```python
from build123d import *

# Parameters (mm, degrees)
F3_R     = 2.5
F4_DEPTH = 76.2


with BuildPart() as f2:
    # F0 (on Front) → F2 (revolve)
    with BuildSketch(Plane.XZ):
        with BuildLine():
            Line((-42, 11.43), (-42, 0))
            Line((-42, 0), (-40, 0))
            Line((-40, 0), (-40, 11.43))
            ThreePointArc((-40, 11.43), (-40.957761, 13.742239), (-43.27, 14.7))
            Line((-43.27, 14.7), (-46, 14.7))
            Line((-46, 14.7), (-46, 94.7))
            Line((-46, 94.7), (-4, 94.7))
            Line((-4, 94.7), (-4, 93.2))
            Line((-4, 93.2), (-4.4, 93.2))
            Line((-4.4, 93.2), (-4, 89.7))
            Line((-4, 89.7), (-4.4, 89.7))
            Line((-4.4, 89.7), (-4, 86.2))
            Line((-4, 86.2), (-2.5, 86.2))
            Line((-2.5, 86.2), (-2.5, 96.7))
            Line((-2.5, 96.7), (-47.365, 96.7))
            ThreePointArc((-47.365, 96.7), (-47.814013, 96.514013), (-48, 96.065))
            Line((-48, 96.065), (-48, 13.97))
            ThreePointArc((-48, 13.97), (-47.628026, 13.071974), (-46.73, 12.7))
            Line((-46.73, 12.7), (-43.27, 12.7))
            ThreePointArc((-43.27, 12.7), (-42.371974, 12.328026), (-42, 11.43))
        make_face()
    revolve(axis=Axis((0, 0, 51.843766), (0, 0, 1)))

    # F3 (on Front) → F4 (cut)
    with BuildSketch(Plane.XZ):
        with Locations((6.35, 43.18)):
            Circle(F3_R)
    extrude(amount=F4_DEPTH, mode=Mode.SUBTRACT)

    # F7 (on offset) → F8 (revolve)
    with BuildSketch(Plane.YZ.offset(6.35)):
        Polygon((-42.69981, 47.18), (-46.19981, 47.18), (-46.19981, 45.68), (-35.69981, 45.68), (-35.69981, 47.18), (-39.19981, 47.18), align=None)
        Polygon((-42.69981, 47.58), (-42.69981, 47.18), (-39.19981, 47.18), align=None)
        Polygon((-39.19981, 47.58), (-39.19981, 47.18), (-35.69981, 47.18), align=None)
    revolve(axis=Axis((6.35, -16.508139, 43.18), (0, 1, 0)))


solid = f2.part
```
Check sheet for the modelled part. Datum: model origin and axes. Units: mm. A direction names the side the tool comes from. Give positions to 0.01 mm unless a question says otherwise; leave off trailing zeros. Loops run counter-clockwise (first coordinate to the right, second up) from the corner with the lowest first, then second, coordinate; pieces in that order, holes last. Notation, with made-up numbers: M 45,61.25 L 70,61.25 A31 cw 70,97.25 Z; hole C -28,37.5 d10. An arc over 180 degrees is marked long. Answer in a Markdown table with one row per item.
1) Mould release check, pull along Y, two halves, no side actions. Record for faces 1 (the face through (0.867, 3.905, 93.94)), 2 (the face through (-37.1, 15.4, 0)), 3 (the face through (10.405, 46.859, 54.443)): released by +Y, released by -Y, zero draft, split by the parting line, or undercut.
Solutions:
| item | result |
|---|---|
| face 1 | undercut |
| face 2 | zero draft |
| face 3 | split by the parting line |
2) Cross-section at A-A (z = 75). Enter the section's corners in (x, y).
Solutions:
| item | result |
|---|---|
| outline | C 0,0 d96; hole C 0,0 d92 |
3) Cross-section at B-B (z = 43.18). Enter the section's corners in (x, y), plus the area to 3 significant figures.
Solutions:
| item | result |
|---|---|
| outline | M 1.95,-42.7 L 2.35,-42.7 L 2.35,-45.94 A46 cw long 10.35,-44.82 L 10.35,-42.7 L 10.75,-42.7 L 10.35,-39.2 L 10.75,-39.2 L 10.35,-35.7 L 8.85,-35.7 L 8.85,-47.18 A48 ccw long 3.85,-47.85 L 3.85,-35.7 L 2.35,-35.7 L 1.95,-39.2 L 2.35,-39.2 Z |
| area | 613 mm^2 |
4) Thickness scan on line 1 (Y direction, x = 0, z = 93.25); line 2 (Y direction, x = 0, z = 47.5). Record the ranges inside material, lowest first.
Solutions:
| item | result |
|---|---|
| line 1 | y = -48 to -46, -4 to -2.5, 2.5 to 4, 46 to 48 |
| line 2 | y = -48 to -46, 46 to 48 |
5) Tool access check on faces 4 (the face through (7.599, -37.085, 47.146)), 5 (the face through (-2, -2, 86.2)), 6 (the face through (10, -1, 96.7)). Record the directions out of +Z, -Z, +X, -X, +Y, -Y that give a thin tool (end or side, any length) a straight path to the whole face; none if there is none.
Solutions:
| item | result |
|---|---|
| face 4 | none |
| face 5 | -Z |
| face 6 | +Z, +X, -X, +Y, -Y |
6) Depth check by flat-ended pin: pin 1 (4.5 mm diameter, centred on x = 6, z = 43.5, fed in from -Y); pin 2 (10 mm diameter, centred on y = -29.5, z = 41, fed in from +X); pin 3 (1 mm diameter, centred on x = -15, z = 38, fed in from -Y). Enter the tip coordinate at first touch or a pass-through.
Solutions:
| item | result |
|---|---|
| pin 1 | stops at y = -47.85 |
| pin 2 | stops at x = 41.28 |
| pin 3 | stops at y = -45.76 |
